Part model, mm, in its own coordinate system. A direction names the side the tool comes from. Coordinates: 2 decimals unless noted, no trailing zeros. Write each loop counter-clockwise with the first axis right and the second up, starting at its lowest first coordinate (ties: lowest second). Pieces come first, ordered by that corner, then holes. Notation, with made-up numbers: (69, 29.25) -> (101, 29.25) arc R24 ccw to (101, 45.25) -> close; hole circle Ø2 at (44, 14). An arc over 180 degrees is marked (long way). One line per question, with ' | ' between items. Start each with the question number.
Item 1: Saw through at B-B (y = -8.5). List the corners of the cut face in (x, z) (3 decimals), and give its area (3 significant figures).
Item 2: Pin check, flat tips, straight feed: pin 1 (8 mm diameter, centred on y = 40.5, z = -11, fed in from +X); pin 2 (4 mm diameter, centred on y = 22.5, z = 7.5, fed in from +X); pin 3 (10 mm diameter, centred on x = 25, z = 11, fed in from +Y). Stop position of each tip, or through.
Item 3: Probe probe 1 along Y at (x, z) = (0, -7.9); probe 2 along Z at (x, y) = (13, 14.5) (3 decimals); probe 3 along Z at (x, y) = (-1.5, -12.5) (3 decimals). List the from-to ranges inside material, lowest first. Write a range as [from, to].
Item 4: 3-axis set-ups, long thin cutter, end or side, ignore diameter. For faces 1 (the cylindrical face through (-0.041, 29.917, -13.959)), 2 (the cylindrical face through (-1.32, 50.47, -9.41)), 3 (the flat face through (19.3, 6.9, 14)), 4 (the flat face through (-19.3, 6.9, -14)), 5 (the cylindrical face through (37.9, -15.3, 13.99)): which of +Z, -Z, +X, -X, +Y, -Y reach the whole face in a straight line?
Item 5: Saw through at A-A (z = -8.5). List the corners of the cut face in (x, y), and give its area (3 significant figures).
Item 6: Two-plate mould, pull along X, no slides. Class faces 6 (the flat face through (6, 21, 5.75)), 7 (the flat face through (1, -16.288, 0)), 8 (the cylindrical face through (-0.8, 16.7, -9.8)), 9 (the flat face through (-18.84, 7.5, 13.96)): pulls with the +X half, pulls with the -X half, needs draft (parallel to the pull), parting line crosses it, or undercut.
Item 7: Saw through at D-D (z = 2.5). List the corners of the cut face in (x, y).
Autodesk Inventor part; units mm, degrees
ref_plane "YZ Plane" through (0, 0, 0) normal (1, 0, 0) x (0, 1, 0)
ref_plane "XY Plane" through (0, 0, 0) normal (0, 0, 1) x (1, 0, 0)
sketch "Sketch1" plane through (0, 0, 0) normal (1, 0, 0) x (0, 1, 0)
  line L0 (-12.5, -12) -> (-9.5, -12)
  line L1 (-9.5, 12) -> (-12.5, 12)
  line L2 (-12.5, 12) -> (-12.5, -12)
  line L3 (-12.5, -12) -> (12.5, 12) construction
  line L4 (12.5, -12) -> (-12.5, 12) construction
  line L5 (20.5, 5.75) -> (-9.5, 5.75)
  line L6 (20.5, -6.75) -> (-9.5, -6.75)
  line L7 (20.5, 5.75) -> (20.5, -6.75)
  line L8 (-9.5, 12) -> (-9.5, 5.75)
  line L9 (-9.5, -6.75) -> (-9.5, -12)
  point P0 (0, 0)
  dimension "d0" = 25
  dimension "d2" = 6.25
  dimension "d3" = 12.5
  dimension "d5" = 24
  dimension "d7" = 3
  dimension "d8" = 3
  dimension "d9" = 30
revolve "Revolution1" add sketch "Sketch1" angle 360 about axis through (0, 20.5, 5.75) along (0, 0, -1)
ref_plane "Work Plane1" through (0, -14.2875, 0) normal (0, 1, 0) x (-1, 0, 0)
sketch "Sketch2" plane through (0, -14.2875, 0) normal (0, 1, 0) x (-1, 0, 0)
  line L0 (38.8032, 14.945) -> (-38.8032, 14.945)
  line L1 (-38.8032, 14.945) -> (-38.8032, -14.945)
  line L2 (-38.8032, -14.945) -> (38.8032, -14.945)
  line L3 (38.8032, -14.945) -> (38.8032, 14.945)
  line L4 (38.8032, 14.945) -> (-38.8032, -14.945) construction
  line L5 (-38.8032, 14.945) -> (38.8032, -14.945) construction
  point P0 (0, 0)
extrude "Extrusion1" add sketch "Sketch2" against normal blind 2
fillet "Fillet1" radius 3.175 4 edges at (-38.8032, -15.2875, 14.945) (-38.8032, -15.2875, -14.945) (38.8032, -15.2875, 14.945) (38.8032, -15.2875, -14.945)
sketch "Sketch3" plane through (-35.6282, -14.2875, 14.945) normal (0, 0, 1) x (1, 0, 0)
  line L0 (71.2564, 0) -> (74.4314, 0)
  line L1 (71.2564, 0) -> (38.1431, 42.9682)
  line L2 (0, -2) -> (0, 0)
  line L3 (33.1133, 42.9682) -> (0, 0)
  line L4 (0, 0) -> (71.2564, 0)
  arc A0 (38.1431, 42.9682) -> (33.1133, 42.9682) centre (35.6282, 41.0302) ccw
  point P0 (35.6282, 14.2875)
  dimension "d14" = 3.175
extrude "Extrusion2" add sketch "Sketch3" against normal blind 2
mirror "Mirror1" about plane through (0, 0, 0) normal (0, 0, 1) of "Extrusion2"
sketch "Sketch4" plane through (-35.6282, -16.2875, 14.945) normal (0, 0, 1) x (1, 0, 0)
  circle A0 centre (35.6282, 36.7875) radius 30
  circle A1 centre (35.6282, 36.7875) radius 3.8819
  point P0 (35.6282, 16.2875)
extrude "Extrusion3" add sketch "Sketch4" against normal blind 28.9875 contours A1
properties part number "roller_coaster_wheel" material "Iron, Gray"
From the geometry:
1) outline: (-31.168, -14.945) -> (31.168, -14.945) -> (31.168, -12.945) -> (-31.168, -12.945) -> close; (-31.168, 12.945) -> (31.168, 12.945) -> (31.168, 14.945) -> (-31.168, 14.945) -> close; (-15.748, -12) -> (-7.681, -12) -> (-7.681, -6.75) -> (7.681, -6.75) -> (7.681, -12) -> (15.748, -12) -> (15.748, 12) -> (7.681, 12) -> (7.681, 5.75) -> (-7.681, 5.75) -> (-7.681, 12) -> (-15.748, 12) -> close | area: 829 mm2
2) pin 1: x = 28.86 | pin 2: x = 33 | pin 3: y = 46.75
3) probe 1: [-16.29, -14.29], [-12.5, -9.5], [16.62, 24.38], [50.5, 53.5] | probe 2: [-14.945, -12.945], [-6.75, 5.75], [12.945, 14.945] | probe 3: [-14.945, -12.945], [12.945, 14.945]
4) face 1: -Z, +Y | face 2: none | face 3: +Z, +X, +Y | face 4: -Z, -X, +Y | face 5: +Z, +X, +Y, -Y
5) outline: (-38.8, -16.29) -> (38.8, -16.29) -> (38.8, -14.29) -> (-38.8, -14.29) -> close; circle Ø66 at (0, 20.5); circle Ø7.76 at (0, 20.5); hole circle Ø60 at (0, 20.5) | area: 796 mm2
6) face 6: undercut | face 7: needs draft | face 8: undercut | face 9: pulls with the -X half
7) outline: (-38.8, -16.29) -> (38.8, -16.29) -> (38.8, -14.29) -> (-38.8, -14.29) -> close; circle Ø66 at (0, 20.5)
